from build123d import *

# Parameters (mm, degrees)
BOSS_EXTRUDE1_DEPTH     = 2.286
SKETCH2_R               = 2.032
SKETCH2_R_2             = 3.81
CUT_EXTRUDE1_DEPTH      = 1
CUT_EXTRUDE1_DEPTH_BACK = 3.286
FILLET1_R               = 2.54
FILLET2_R               = 2.54


with BuildPart() as part:
    # Sketch1 → Boss-Extrude1 (new body)
    with BuildSketch(Plane(origin=(0, 0, 0), x_dir=(1, 0, 0), z_dir=(0, 1, 0))):
        with BuildLine():
            ThreePointArc((25.4, -25.4), (12.7, -12.7), (0, -25.4))
            Line((0, -25.4), (25.4, -25.4))
        make_face()
        with BuildLine():
            Line((25.4, -25.4), (0, -25.4))
            ThreePointArc((0, -25.4), (12.7, -38.1), (25.4, -25.4))
        make_face()
        with BuildLine():
            Line((25.4, 0), (0, 0))
            Line((0, 0), (0, -25.4))
            ThreePointArc((0, -25.4), (12.7, -12.7), (25.4, -25.4))
            Line((25.4, -25.4), (25.4, 0))
        make_face()
    extrude(amount=BOSS_EXTRUDE1_DEPTH)

    # Sketch2 → Cut-Extrude1 (cut, two sides)
    with BuildSketch(Plane(origin=(0, 2.286, 0), x_dir=(1, 0, 0), z_dir=(0, 1, 0))) as cut_extrude1_sk:
        with Locations((12.7, -12.7)):
            Circle(SKETCH2_R)
        with Locations((12.7, -31.75)):
            Circle(SKETCH2_R_2)
    extrude(amount=CUT_EXTRUDE1_DEPTH, mode=Mode.SUBTRACT)
    extrude(cut_extrude1_sk.sketch, amount=-CUT_EXTRUDE1_DEPTH_BACK, mode=Mode.SUBTRACT)

    # Fillet1
    fillet1_edges = [part.edges().sort_by_distance(p)[0] for p in [
        (0, 1.143, 0),
    ]]
    fillet(fillet1_edges, radius=FILLET1_R)

    # Fillet2
    fillet2_edges = [part.edges().sort_by_distance(p)[0] for p in [
        (25.4, 1.143, 0),
    ]]
    fillet(fillet2_edges, radius=FILLET2_R)


solid = part.part
Verification items for the finished model (mm, model axes). Round coordinates to 2 decimals unless told otherwise and drop trailing zeros. Order: outer loops, then holes, each group sorted by start corner. A loop starts at its lowest first (then second) coordinate and runs counter-clockwise, first axis right, second up.
1. Section check A-A on x = 12.7. Record the cut outline in (y, z), then the cut area to 3 significant figures.
Final values:
outline: (0, 0) - (2.29, 0) - (2.29, 10.67) - (0, 10.67) - close; (0, 14.73) - (2.29, 14.73) - (2.29, 27.94) - (0, 27.94) - close; (0, 35.56) - (2.29, 35.56) - (2.29, 38.1) - (0, 38.1) - close
area: 60.4 mm2
2. Section check D-D on z = 35. Record the cut outline in (x, y).
Final values:
outline: (4.39, 0) - (10.71, 0) - (10.71, 2.29) - (4.39, 2.29) - close; (14.69, 0) - (21.01, 0) - (21.01, 2.29) - (14.69, 2.29) - close
3. Section check B-B on z = 12.7. Record the cut outline in (x, y).
Final values:
outline: (0, 0) - (10.67, 0) - (10.67, 2.29) - (0, 2.29) - close; (14.73, 0) - (25.4, 0) - (25.4, 2.29) - (14.73, 2.29) - close
4. Section check C-C on y = 0.45. Record the cut outline in (x, z).
Final values:
outline: (0, 2.54) arc R2.54 ccw to (2.54, 0) - (22.86, 0) arc R2.54 ccw to (25.4, 2.54) - (25.4, 25.4) arc R12.7 ccw to (0, 25.4) - close; hole circle Ø7.62 at (12.7, 31.75); hole circle Ø4.06 at (12.7, 12.7)
5. Thickness scan on L1, parallel to Z at x = 12.7, y = 0.85; L2, parallel to X at y = 1.7, z = 12.7; L3, parallel to Z at x = 11, y = 1.4. Record the ranges inside material, lowest first.
Final values:
L1: z = 0 to 10.67, 14.73 to 27.94, 35.56 to 38.1
L2: x = 0 to 10.67, 14.73 to 25.4
L3: z = 0 to 11.59, 13.81 to 28.34, 35.16 to 37.99
6. Release check for a two-part mould opening along Z. For faces 1 (the cylindrical face through (0.724, 1.159, 0.764)), 2 (the cylindrical face through (11.09, 1.16, 13.94)), 3 (the cylindrical face through (11.87, 1.16, 35.47)), 4 (the flat face through (13, 0, 19)) record: +Z half, -Z half, draft (parallel to the pull), parting line (faces both ways), or undercut.
Final values:
face 1: -Z half
face 2: undercut
face 3: undercut
face 4: draft
7. Go/stop test with flat-tipped pins: P1, Ø5, axis at x = 17, z = 23.5, coming from the -Y side; P2, Ø3.5, axis at x = 12.7, z = 12.7, coming from the -Y side. Record where each tip stops, or that it passes through.
Final values:
P1: stops at y = 0
P2: passes through
